CAD build for the part. Positions are in the model's coordinates, mm. Round coordinates to 2 decimals unless told otherwise and drop trailing zeros. Loops run counter-clockwise (first coordinate to the right, second up) from the corner with the lowest first, then second, coordinate; pieces in that order, holes last. Notation, with made-up numbers: M 75,36.25 L 121,36.25 A19 cw 121,52.25 Z; hole C 66.5,2.5 d8. An arc over 180 degrees is marked long. Put each result on its own line as item: value. Start each with the question number.
from build123d import *

# Parameters (mm, degrees)
SKETCH_1_W          = 80
SKETCH_1_H          = 31.819805153
SKETCH_1_H_2        = 20
EXTRUDE_1_DEPTH     = 1
CUT_EXTRUDE_1_DEPTH = 10
CHAMFER_1_SIZE      = 10
SKETCH_4_R          = 1.6
SKETCH_4_R_2        = 2.1
CUT_EXTRUDE_2_DEPTH = 10


with BuildPart() as part:
    # 草图1 → 凸台-拉伸1 (new body)
    with BuildSketch(Plane(origin=(0, 0, 0), x_dir=(1, 0, 0), z_dir=(0, 1, 0))):
        with Locations((40, 15.909902577)):
            Rectangle(SKETCH_1_W, SKETCH_1_H)
        with Locations((40, -10)):
            Rectangle(SKETCH_1_W, SKETCH_1_H_2)
    extrude(amount=EXTRUDE_1_DEPTH)

    # 草图3 → 切除-拉伸1 (cut)
    with BuildSketch(Plane(origin=(0, 1, 0), x_dir=(1, 0, 0), z_dir=(0, 1, 0))):
        Polygon((80, -20), (80, 40), (20, -20), align=None)
    extrude(amount=-CUT_EXTRUDE_1_DEPTH, mode=Mode.SUBTRACT)

    # 倒角1
    chamfer_1_edges = [part.edges().sort_by_distance(p)[0] for p in [
        (0, 0.5, 20),
        (71.819805153, 0.5, -31.819805153),
        (0, 0.5, -31.819805153),
    ]]
    chamfer(chamfer_1_edges, length=CHAMFER_1_SIZE)

    # 草图4 → 切除-拉伸2 (cut)
    with BuildSketch(Plane(origin=(0, 1, 0), x_dir=(1, 0, 0), z_dir=(0, 1, 0))):
        with Locations(Location((5, 15.909902577, 0), (0, 0, 270))):
            Circle(SKETCH_4_R)
        with Locations(Location((5, -4.090097423, 0), (0, 0, 270))):
            Circle(SKETCH_4_R)
        with Locations(Location((25, 19.819805153, 0), (0, 0, 270))):
            Circle(SKETCH_4_R_2)
    extrude(amount=-CUT_EXTRUDE_2_DEPTH, mode=Mode.SUBTRACT)


solid = part.part
(1) Cut at C-C on y = 0.6. List the corners of the cut face in (x, z).
(2) Cut at D-D on x = 5. List the corners of the cut face in (y, z).
(3) Cut at B-B on z = -19. List the corners of the cut face in (x, y).
(4) Mould opens along Z. For faces 1 (the flat face through (42.7, 0.5, -2.7)), 2 (the flat face through (63.305, 0.493, -28.235)), 3 (the cylindrical face through (4.39, 0.51, 5.57)) say: +Z half, -Z half, draft (parallel to the pull), parting line (faces both ways), or undercut.
(5) Cut at A-A on x = 25. List the corners of the cut face in (y, z).
(6) Flat gauge pin, fed straight in: pin 1 Ø12 at (x, z) = (55, -11) entering from -Y. Where does the tip first touch, or does it go through?
(7) Drill centre lines: line 1 along X through (y, z) = (0.8, -20); line 2 along X through (y, z) = (0.65, -17); line 3 along X through (y, z) = (0.9, -29.5). Where is each one in solid material? Low to high.
Taken from the geometry:
1. outline: M 0,-21.82 L 10,-31.82 L 61.82,-31.82 L 64.75,-24.75 L 20,20 L 10,20 L 0,10 Z; hole C 5,-15.91 d3.2; hole C 5,4.09 d3.2; hole C 25,-19.82 d4.2
2. outline: M 0,-26.82 L 1,-26.82 L 1,-17.51 L 0,-17.51 Z; M 0,-14.31 L 1,-14.31 L 1,2.49 L 0,2.49 Z; M 0,5.69 L 1,5.69 L 1,15 L 0,15 Z
3. outline: M 0,0 L 23.07,0 L 23.07,1 L 0,1 Z; M 26.93,0 L 59,0 L 59,1 L 26.93,1 Z
4. face 1: +Z half
4. face 2: -Z half
4. face 3: undercut
5. outline: M 0,-31.82 L 1,-31.82 L 1,-21.92 L 0,-21.92 Z; M 0,-17.72 L 1,-17.72 L 1,15 L 0,15 Z
6. pin 1: y = 0
7. line 1: 0 to 22.91, 27.09 to 60
7. line 2: 0 to 3.83, 6.17 to 57
7. line 3: 7.68 to 62.78
